Geometry: see drawing. Coordinates: mm, zero at the bounding-box minimum. Give positions to 0.01 mm unless a question says otherwise; leave off trailing zeros. Write each loop counter-clockwise with the first axis right and the second up, starting at its lowest first coordinate (ties: lowest second). Pieces come first, ordered by that corner, then holes. Notation, with made-up numbers: (73, 41.25) - (125, 41.25) arc R21 cw to (125, 48.25) - close; hole circle Ø11 at (-12.5, 9). An arc over 180 degrees is marked (long way). Return JSON: item names as keys, results as strings.
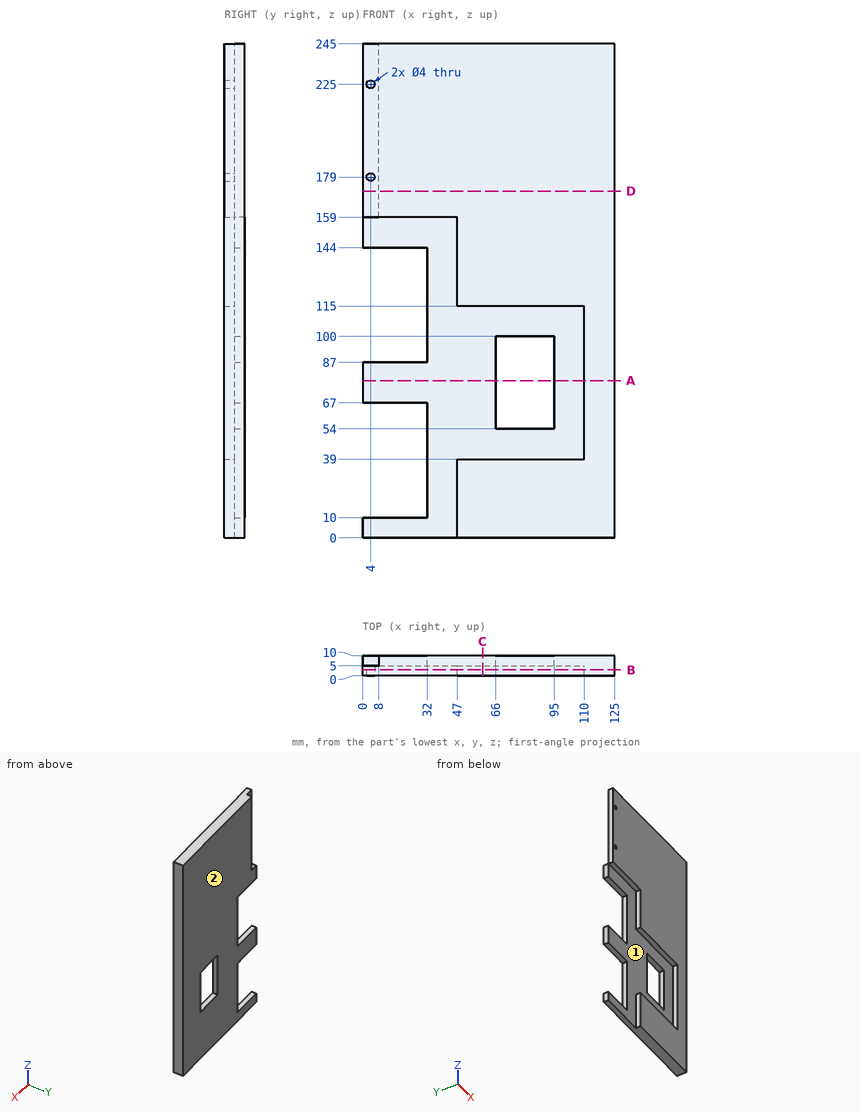
Q1. Material intervals for probe 1 along Z at (x, y) = (4, 2.25); probe 2 along X at (y, z) = (1.8, 179); probe 3 along Z at (x, y) = (91, 3.5), sorted ascending. Write a range as [from, to].
Answer key:
{"probe 1": "z = [159, 177], [181, 223], [227, 245]", "probe 2": "x = [0, 2], [6, 125]", "probe 3": "z = [0, 39], [115, 245]"}
Q2. Section query C-C, the plane x = 59.5. Return the cut outline in (y, z).
Answer key:
{"outline": "(0, 0) - (10, 0) - (10, 245) - (0, 245) - (0, 115) - (5, 115) - (5, 39) - (0, 39) - close"}
Q3. Pin query (flat end, axial travel): P1, Ø1.5, axis at y = 6.5, z = 209.5, coming from the -X side; P2, Ø4, axis at y = 2.5, z = 58.5, coming from the -X side; P3, Ø2.5, axis at x = 15, y = 1.5, coming from the -Z side. Return the tip coordinate at first contact, or that it passes through.
Answer key:
{"P1": "stops at x = 8", "P2": "stops at x = 110", "P3": "stops at z = 159"}
Q4. Section query B-B, the plane y = 3. Return the cut outline in (x, z), plus the area to 3 significant figures.
Answer key:
{"outline": "(0, 159) - (47, 159) - (47, 115) - (110, 115) - (110, 39) - (47, 39) - (47, 0) - (125, 0) - (125, 245) - (0, 245) - close; hole circle Ø4 at (4, 179); hole circle Ø4 at (4, 225)", "area": "18,300 mm^2"}
Q5. Mould query, pull axis Z, two halves, no side actions, for the marked faces 1 and 2. Classes: pulls with the +Z half, pulls with the -Z half, needs draft (parallel to the pull), parting line crosses it, or undercut.
Answer key:
{"face 1": "undercut", "face 2": "needs draft"}
Q6. Section query D-D, the plane z = 172. Return the cut outline in (x, y).
Answer key:
{"outline": "(0, 0) - (125, 0) - (125, 10) - (8, 10) - (8, 5) - (0, 5) - close"}
Q7. Section query A-A, the plane z = 78. Return the cut outline in (x, y).
Answer key:
{"outline": "(0, 5) - (66, 5) - (66, 10) - (0, 10) - close; (95, 5) - (110, 5) - (110, 0) - (125, 0) - (125, 10) - (95, 10) - close"}
